from build123d import *

# Parameters (mm, degrees)
SKETCH_1_W          = 55
SKETCH_1_H          = 31
SKETCH_1_W_2        = 52
SKETCH_1_H_2        = 27
EXTRUDE_1_DEPTH     = 10
SKETCH_2_W          = 55
SKETCH_2_H          = 31
EXTRUDE_2_DEPTH     = 1.6
CUT_EXTRUDE_1_REACH = 66.192
SKETCH_3_W          = 31
SKETCH_3_H          = 20
SKETCH_4_W          = 52
SKETCH_4_H          = 27
SKETCH_4_W_2        = 35
SKETCH_4_H_2        = 24
EXTRUDE_3_DEPTH     = 1.5
SKETCH_5_W          = 15
SKETCH_5_H          = 2
CUT_EXTRUDE_2_DEPTH = 1.5
SKETCH_7_W          = 9.5
SKETCH_7_H          = 9.6
CUT_EXTRUDE_4_DEPTH = 5
SKETCH_8_W          = 1
SKETCH_8_H          = 9.6
CUT_EXTRUDE_5_DEPTH = 1.5
SKETCH_9_W          = 1
SKETCH_9_H          = 13
CUT_EXTRUDE_6_DEPTH = 5.5
SKETCH_10_R         = 1.75
CUT_EXTRUDE_7_DEPTH = 64.704395453
FILLET_1_R          = 3
FILLET_2_R          = 4.5
FILLET_3_R          = 1.5
FILLET_4_R          = 1.5
CHAMFER_1_SIZE      = 0.7


with BuildPart() as part:
    # 草图1 → 凸台-拉伸1 (new body)
    with BuildSketch(Plane.XY):
        with Locations((27.5, -15.5)):
            Rectangle(SKETCH_1_W, SKETCH_1_H)
        with Locations((28, -15.5)):
            Rectangle(SKETCH_1_W_2, SKETCH_1_H_2, mode=Mode.SUBTRACT)
    extrude(amount=EXTRUDE_1_DEPTH)

    # 草图2 → 凸台-拉伸2 (add)
    with BuildSketch(Plane.XY.offset(10)):
        with Locations((27.5, -15.5)):
            Rectangle(SKETCH_2_W, SKETCH_2_H)
    extrude(amount=EXTRUDE_2_DEPTH)

    # 草图3 → 切除-拉伸1 (cut, up to next)
    with BuildSketch(Plane.XY.offset(11.6), mode=Mode.PRIVATE) as cut_extrude_1_sk1:
        with Locations((28, -15)):
            Rectangle(SKETCH_3_W, SKETCH_3_H)
    cut_extrude_1_tool1 = extrude(cut_extrude_1_sk1.sketch, amount=-CUT_EXTRUDE_1_REACH, mode=Mode.PRIVATE) & part.part
    add(cut_extrude_1_tool1.solids().sort_by_distance((28, -15, 11.6))[0], mode=Mode.SUBTRACT)

    # 草图4 → 凸台-拉伸3 (add)
    with BuildSketch(Plane(origin=(0, 0, 10), x_dir=(-1, 0, 0), z_dir=(0, 0, -1))):
        with Locations((-28, -15.5)):
            Rectangle(SKETCH_4_W, SKETCH_4_H)
        with Locations((-28, -15)):
            Rectangle(SKETCH_4_W_2, SKETCH_4_H_2, mode=Mode.SUBTRACT)
    extrude(amount=EXTRUDE_3_DEPTH)

    # 草图5 → 切除-拉伸2 (cut)
    with BuildSketch(Plane(origin=(0, 0, 8.5), x_dir=(-1, 0, 0), z_dir=(0, 0, -1))):
        with Locations((-28, -28)):
            Rectangle(SKETCH_5_W, SKETCH_5_H)
    extrude(amount=-CUT_EXTRUDE_2_DEPTH, mode=Mode.SUBTRACT)

    # 草图7 → 切除-拉伸4 (cut)
    with BuildSketch(Plane.XY.offset(11.6)):
        with Locations((4.75, -15.5)):
            Rectangle(SKETCH_7_W, SKETCH_7_H)
    extrude(amount=-CUT_EXTRUDE_4_DEPTH, mode=Mode.SUBTRACT)

    # 草图8 → 切除-拉伸5 (cut)
    with BuildSketch(Plane(origin=(0, 0, 8.5), x_dir=(-1, 0, 0), z_dir=(0, 0, -1))):
        with Locations((-10, -15.5)):
            Rectangle(SKETCH_8_W, SKETCH_8_H)
    extrude(amount=-CUT_EXTRUDE_5_DEPTH, mode=Mode.SUBTRACT)

    # 草图9 → 切除-拉伸6 (cut)
    with BuildSketch(Plane(origin=(0, 0, 0), x_dir=(-1, 0, 0), z_dir=(0, 0, -1))):
        with Locations((-54.5, -15.8)):
            Rectangle(SKETCH_9_W, SKETCH_9_H)
    extrude(amount=-CUT_EXTRUDE_6_DEPTH, mode=Mode.SUBTRACT)

    # 草图10 → 切除-拉伸7 (cut, through all)
    with BuildSketch(Plane(origin=(0, 0, 8.5), x_dir=(-1, 0, 0), z_dir=(0, 0, -1))):
        with Locations((-50.6, -5.4)):
            Circle(SKETCH_10_R)
        with Locations((-5.388, -5.4)):
            Circle(SKETCH_10_R)
        with Locations((-5.388, -25.6)):
            Circle(SKETCH_10_R)
        with Locations((-50.6, -25.6)):
            Circle(SKETCH_10_R)
    extrude(amount=-CUT_EXTRUDE_7_DEPTH, mode=Mode.SUBTRACT)

    # 圆角1
    fillet_1_edges = [part.edges().sort_by_distance(p)[0] for p in [
        (54, -2, 4.25),
        (2, -2, 4.25),
        (54, -29, 4.25),
        (2, -29, 4.25),
    ]]
    fillet(fillet_1_edges, radius=FILLET_1_R)

    # 圆角2
    fillet_2_edges = [part.edges().sort_by_distance(p)[0] for p in [
        (0, 0, 5.8),
        (55, 0, 5.8),
        (55, -31, 5.8),
        (0, -31, 5.8),
    ]]
    fillet(fillet_2_edges, radius=FILLET_2_R)

    # 圆角3
    fillet_3_edges = [part.edges().sort_by_distance(p)[0] for p in [
        (1, -10.7, 6.6),
        (1, -20.3, 6.6),
    ]]
    fillet(fillet_3_edges, radius=FILLET_3_R)

    # 圆角4
    fillet_4_edges = [part.edges().sort_by_distance(p)[0] for p in [
        (0, -7.6, 11.6),
        (27.5, 0, 11.6),
        (27.5, -31, 11.6),
        (55, -15.5, 11.6),
        (53.681980515, -1.318019485, 11.6),
        (53.681980515, -29.681980515, 11.6),
        (1.318019485, -29.681980515, 11.6),
        (1.318019485, -1.318019485, 11.6),
        (0, -23.4, 11.6),
    ]]
    fillet(fillet_4_edges, radius=FILLET_4_R)

    # 倒角1
    chamfer_1_edges = [part.edges().sort_by_distance(p)[0] for p in [
        (52.35, -25.6, 11.6),
        (7.138, -25.6, 11.6),
        (7.138, -5.4, 11.6),
        (52.35, -5.4, 11.6),
    ]]
    chamfer(chamfer_1_edges, length=CHAMFER_1_SIZE)


solid = part.part
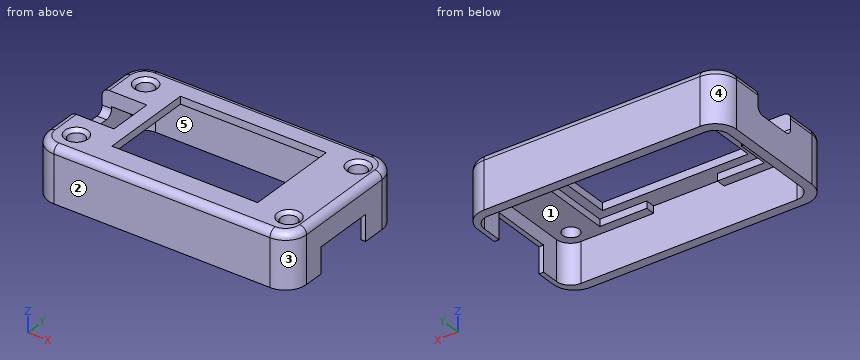
Build history of the part. All positions in model axes, mm. Face numbers are marked on the shaded views. A direction names the side the tool comes from. Round coordinates to 2 decimals unless told otherwise and drop trailing zeros. Write each loop counter-clockwise with the first axis right and the second up, starting at its lowest first coordinate (ties: lowest second). Pieces come first, ordered by that corner, then holes. Notation, with made-up numbers: (21, 26) - (54, 26) arc R19 cw to (54, 54) - close; hole circle Ø6 at (60.5, 6). An arc over 180 degrees is marked (long way). One line per question, with ' | ' between items.
1. Band-saw the part on A-A, the plane y = -14.5. Write the cut outline in (x, z).
Results are:
outline: (0, 0) - (2, 0) - (2, 6.6) - (0, 6.6) - close; (9.5, 10) - (12.5, 10) - (12.5, 11.6) - (9.5, 11.6) - close; (43.5, 10) - (45.5, 10) - (45.5, 8.5) - (54, 8.5) - (54, 5.5) - (55, 5.5) - (55, 10.1) arc R1.5 ccw to (53.5, 11.6) - (43.5, 11.6) - close
2. Drop flat-ended pins along their axis: pin 1 Ø2 at (x, y) = (13, -16.5) entering from -Z; pin 2 Ø13.5 at (x, y) = (19.5, -14.5) entering from -Z; pin 3 Ø0.5 at (x, z) = (54.5, 4) entering from +Y; pin 4 Ø0.8 at (y, z) = (-27.5, 9) entering from +X. Give the stop position or say it passes through.
Results are:
pin 1: z = 10 | pin 2: through | pin 3: y = -2.01 | pin 4: x = 54.96
3. Band-saw the part on D-D, the plane x = 41. Write the cut outline in (y, z), and give its area (3 significant figures).
Results are:
outline: (-31, 0) - (-29, 0) - (-29, 8.5) - (-27, 8.5) - (-27, 10) - (-25, 10) - (-25, 11.6) - (-29.5, 11.6) arc R1.5 ccw to (-31, 10.1) - close; (-5, 10) - (-3, 10) - (-3, 8.5) - (-2, 8.5) - (-2, 0) - (0, 0) - (0, 10.1) arc R1.5 ccw to (-1.5, 11.6) - (-5, 11.6) - close | area: 61.1 mm^2
4. Drill centre lines: line 1 along Y through (x, z) = (50.6, 9.5); line 2 along Y through (x, z) = (29, 1.5); line 3 along Z through (x, y) = (50.5, -13.5). Where is each one in solid material? Low to high. Write a range as from..to.
Results are:
line 1: -31..-27.35, -23.85..-7.15, -3.65..0 | line 2: -31..-29, -2..0 | line 3: 8.5..11.6
5. Mould opens along Y. For the marked faces 3, 4 and 5 say: released by +Y, released by -Y, zero draft, split by the parting line, or undercut.
Results are:
face 3: released by -Y | face 4: released by +Y | face 5: undercut
6. Band-saw the part on C-C, the plane z = 3.75. Write the cut outline in (x, y), and give its area (3 significant figures).
Results are:
outline: (0, -26.5) arc R4.5 ccw to (4.5, -31) - (50.5, -31) arc R4.5 ccw to (55, -26.5) - (55, -22.3) - (54, -22.3) - (54, -26) arc R3 cw to (51, -29) - (5, -29) arc R3 cw to (2, -26) - (2, -5) arc R3 cw to (5, -2) - (51, -2) arc R3 cw to (54, -5) - (54, -9.3) - (55, -9.3) - (55, -4.5) arc R4.5 ccw to (50.5, 0) - (4.5, 0) arc R4.5 ccw to (0, -4.5) - close | area: 278 mm^2
7. Band-saw the part on B-B, the plane x = 25. Write the cut outline in (y, z).
Results are:
outline: (-31, 0) - (-29, 0) - (-29, 10) - (-25, 10) - (-25, 11.6) - (-29.5, 11.6) arc R1.5 ccw to (-31, 10.1) - close; (-5, 10) - (-3, 10) - (-3, 8.5) - (-2, 8.5) - (-2, 0) - (0, 0) - (0, 10.1) arc R1.5 ccw to (-1.5, 11.6) - (-5, 11.6) - close
8. Tool access for the marked faces 1 and 2: list every direction of +Z, -Z, +X, -X, +Y, -Y with a clear straight run to the whole face (end or side of a thin tool).
Results are:
face 1: -Z | face 2: +Z, -Z, +X, -X, -Y
